Work out the finished part from the listing and answer in its coordinate system (mm). Face numbers are marked on the shaded views. A direction names the side the tool comes from. Round coordinates to 2 decimals unless told otherwise and drop trailing zeros. Write each loop counter-clockwise with the first axis right and the second up, starting at its lowest first coordinate (ties: lowest second). Pieces come first, ordered by that corner, then holes. Notation, with made-up numbers: (20.25, 14.25) - (34.25, 14.25) arc R33 cw to (34.25, 48.25) - close; hole circle Ø5 at (89.5, 16). An arc over 180 degrees is marked (long way). Answer as a JSON object with one key per item and string values.
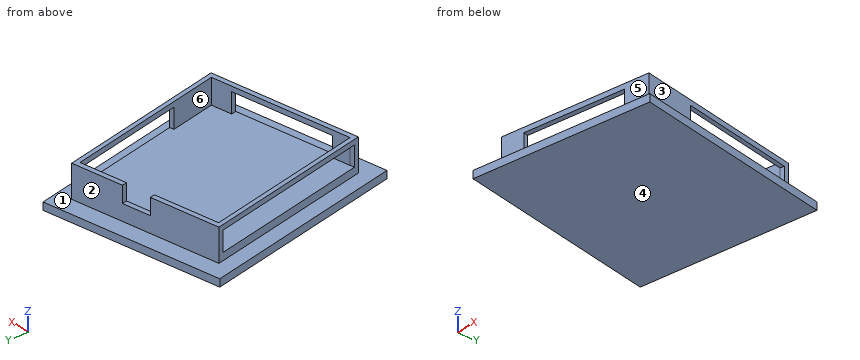
Autodesk Inventor part; units mm, degrees
ref_plane "YZ Plane" through (0, 0, 0) normal (1, 0, 0) x (0, 1, 0)
ref_plane "XZ Plane" through (0, 0, 0) normal (0, 1, 0) x (-1, 0, 0)
ref_plane "XY Plane" through (0, 0, 0) normal (0, 0, 1) x (1, 0, 0)
ref_plane "Work Plane1" through (80.3117, 823.0211, 0) normal (0, 0, 1) x (0.9814259, 0.1918418, 0)
sketch "Sketch1" plane through (80.3117, 823.0211, 0) normal (0, 0, 1) x (0.9814259, 0.1918418, 0)
  line L0 (98.9183, 339.573) -> (44.3184, 339.573)
  line L1 (44.3184, 339.573) -> (44.3184, 276.403)
  line L2 (44.3184, 276.403) -> (98.9183, 276.403)
  line L3 (98.9183, 276.403) -> (98.9183, 339.573)
  line L4 (98.9183, 339.573) -> (44.3184, 276.403)
  line L5 (42.6184, 341.488) -> (100.6184, 341.488)
  line L6 (100.6184, 341.488) -> (100.6184, 274.488)
  line L7 (100.6184, 274.488) -> (42.6184, 274.488)
  line L8 (42.6184, 274.488) -> (42.6184, 341.488)
  line L9 (42.6184, 341.488) -> (100.6184, 274.488) construction
  line L10 (100.6184, 341.488) -> (42.6184, 274.488) construction
  line L11 (98.9183, 339.573) -> (44.3184, 339.573)
  line L12 (44.3184, 339.573) -> (44.3184, 276.403)
  line L13 (44.3184, 276.403) -> (98.9183, 276.403)
  line L14 (98.9183, 276.403) -> (98.9183, 339.573)
  line L15 (98.9183, 339.573) -> (44.3184, 276.403)
  line L16 (42.6184, 341.488) -> (100.6184, 341.488)
  line L17 (100.6184, 341.488) -> (100.6184, 274.488)
  line L18 (100.6184, 274.488) -> (42.6184, 274.488)
  line L19 (42.6184, 274.488) -> (42.6184, 341.488)
  line L20 (42.6184, 341.488) -> (100.6184, 274.488) construction
  line L21 (100.6184, 341.488) -> (42.6184, 274.488) construction
  point P0 (-236.7099, -792.3271)
  point P1 (71.6184, 307.988)
  point P2 (0, 0)
  point P3 (71.6184, 307.988)
  dimension "d0" = 58
  dimension "d1" = 67
  dimension "d2" = 58
  dimension "d3" = 67
sketch "Sketch2" plane through (80.3117, 823.0211, 0) normal (0, 0, 1) x (0.9814259, 0.1918418, 0)
  line L0 (98.9183, 339.573) -> (44.3184, 339.573)
  line L1 (44.3184, 339.573) -> (44.3184, 276.403)
  line L2 (44.3184, 276.403) -> (98.9183, 276.403)
  line L3 (98.9183, 276.403) -> (98.9183, 339.573)
  line L4 (42.6184, 341.488) -> (100.6184, 341.488)
  line L5 (100.6184, 341.488) -> (100.6184, 274.488)
  line L6 (100.6184, 274.488) -> (42.6184, 274.488)
  line L7 (42.6184, 274.488) -> (42.6184, 341.488)
  line L8 (42.6184, 341.488) -> (100.6184, 274.488) construction
  line L9 (100.6184, 341.488) -> (42.6184, 274.488) construction
  line L10 (98.9183, 339.573) -> (44.3184, 339.573)
  line L11 (44.3184, 339.573) -> (44.3184, 276.403)
  line L12 (44.3184, 276.403) -> (98.9183, 276.403)
  line L13 (98.9183, 276.403) -> (98.9183, 339.573)
  line L14 (42.6184, 341.488) -> (100.6184, 341.488)
  line L15 (100.6184, 341.488) -> (100.6184, 274.488)
  line L16 (100.6184, 274.488) -> (42.6184, 274.488)
  line L17 (42.6184, 274.488) -> (42.6184, 341.488)
  line L18 (42.6184, 341.488) -> (100.6184, 274.488) construction
  line L19 (100.6184, 341.488) -> (42.6184, 274.488) construction
  point P0 (-236.7099, -792.3271)
  point P1 (0, 0)
  point P2 (71.6184, 307.988)
  point P3 (0, 0)
  point P4 (71.6184, 307.988)
  dimension "d4" = 58
  dimension "d5" = 67
  dimension "d6" = 58
  dimension "d7" = 67
extrude "Extrusion1" add sketch "Sketch1" along normal blind 10
extrude "Extrusion3" add sketch "Sketch2" against normal blind 3 contours L3 L2 L1 L0 | L4 L5 L6 L7
sketch "Sketch4" plane through (69.4802, 1100.5867, -3) normal (-0.9814259, -0.1918418, 0) x (0, 0, 1)
  line L0 (3, 65.085) -> (13, 65.085)
  line L1 (3, 1.915) -> (13, 1.915)
  line L2 (3, 65.085) -> (11, 65.085)
  line L3 (11, 65.085) -> (11, 1.915)
  line L4 (11, 1.915) -> (3, 1.915)
  line L5 (3, 1.915) -> (3, 65.085)
  point P0 (3, -1066.8151)
  dimension "d14" = 8
extrude "Extrusion4" cut sketch "Sketch4" against normal blind 3
sketch "Sketch5" plane through (126.4029, 1111.7135, -3) normal (0.1918418, -0.9814259, 0) x (0.9814259, 0.1918418, 0)
  line L0 (-56.3, 5) -> (-56.3, 3)
  line L1 (-41.56, 9.2) -> (-44.06, 9.2)
  line L2 (-14.575, 10) -> (-14.575, 9.2)
  line L3 (-9.7, 11) -> (-9.7, 3)
  line L4 (-46.3, 11) -> (-9.7, 11)
  line L5 (-9.7, 3) -> (-46.3, 3)
  line L6 (-58, 3) -> (-1.7, 3)
  line L7 (-46.3, 11) -> (-43.3, 11)
  line L8 (-43.3, 3) -> (-46.3, 3)
  line L9 (-46.3, 11) -> (-49.3, 11)
  line L10 (-49.3, 11) -> (-49.3, 3)
  line L11 (-49.3, 3) -> (-46.3, 3)
  point P0 (-337.3282, 3)
  dimension "d22" = 8
  dimension "d24" = 8
  dimension "d33" = 3
  dimension "d34" = 3
extrude "Extrusion5" cut sketch "Sketch5" against normal blind 3
sketch "Sketch6" plane through (113.5495, 1177.4691, 10) normal (0.9814259, 0.1918418, 0) x (0, 0, -1)
  line L0 (8, -44.46) -> (3, -44.46)
  line L1 (2, -65.085) -> (2, -1.915)
  line L2 (2, -65.085) -> (10, -65.085)
  line L3 (10, -65.085) -> (10, -47.085)
  line L4 (10, -47.085) -> (2, -47.085)
  line L5 (2, -47.085) -> (2, -65.085)
  line L6 (10, -65.085) -> (10, -1.915)
  line L7 (2, -47.085) -> (10, -47.085)
  line L8 (10, -47.085) -> (10, -1.915)
  line L9 (10, -1.915) -> (2, -1.915)
  line L10 (2, -1.915) -> (2, -47.085)
  point P0 (10, -1133.8151)
  dimension "d25" = 8
  dimension "d26" = 18
extrude "Extrusion6" cut sketch "Sketch6" against normal blind 3 contours L1 L9 L6 L4
sketch "Sketch7" plane through (56.9942, 1164.4628, 0) normal (0.1918418, -0.9814259, 0) x (0.9814259, 0.1918418, 0)
  line L0 (28.4907, 10.1469) -> (28.4907, 10.1469)
  line L1 (27, 8) -> (27, 3.4394)
  line L2 (27, 3.4394) -> (38, 3.4394)
  line L3 (38, 3.4394) -> (38, 8)
  line L4 (38, 3.4394) -> (27, 3.4394)
  line L5 (27, 3.4394) -> (27, 13.4394)
  line L6 (27, 13.4394) -> (38, 13.4394)
  line L7 (38, 13.4394) -> (38, 3.4394)
  point P0 (-279.3282, 0)
  point P1 (35.9907, 10.1469)
  dimension "d29" = 11
  dimension "d32" = 10
extrude "Extrusion7" cut sketch "Sketch7" against normal blind 3
sketch "Sketch8" plane through (80.3117, 823.0211, -3) normal (0, 0, -1) x (-0.9814259, -0.1918418, 0)
  line L0 (-42.6184, 341.488) -> (-100.6184, 341.488)
  line L1 (-100.6184, 341.488) -> (-100.6184, 274.488)
  line L2 (-42.6184, 274.488) -> (-42.6184, 341.488)
  line L3 (-100.6184, 274.488) -> (-42.6184, 274.488)
  line L4 (-106.4184, 348.188) -> (-36.8184, 348.188)
  line L5 (-36.8184, 348.188) -> (-36.8184, 267.788)
  line L6 (-36.8184, 267.788) -> (-106.4184, 267.788)
  line L7 (-106.4184, 267.788) -> (-106.4184, 348.188)
  point P0 (236.7099, -792.3271)
  point P1 (-71.6184, 341.488)
  point P2 (-71.6184, 307.988)
extrude "Extrusion8" add sketch "Sketch8" along normal blind 3 contours L2 L3 L1 L0 | L4 L5 L6 L7
properties part number "Syno"
Item 1: A cutting plane is placed at D-D (x = 89). Write down the section's boundary in (y, z), and give its area (3 significant figures).
Results found:
{"outline": "(1097.58, -6) - (1179.5, -6) - (1179.5, -3) - (1172.67, -3) - (1172.67, 3.44) - (1170.72, 3.44) - (1170.72, 0) - (1104.4, 0) - (1104.4, -3) - (1097.58, -3) - close; (1104.4, 8) - (1106.35, 8) - (1106.35, 10) - (1104.4, 10) - close", "area": "461 mm²"}
Item 2: For the marked faces 1, 2 and 3, determine the directions among +Z, -Z, +X, -X, +Y, -Y from which every point of the face is accessible in a straight line to the end or side of a thin tool.
Results found:
{"face 1": "+Z", "face 2": "+Z, -X, +Y", "face 3": "+Z, +X, +Y"}
Item 3: Consider line 1 along Z through (x, y) = (61.5, 1173); line 2 along Z through (x, y) = (82, 1122); line 3 along Y through (x, z) = (76, 8). Determine where each line is inside the solid, lowest interval first.
Results found:
{"line 1": "-6 to -3", "line 2": "-6 to 0", "line 3": "1101.86 to 1103.81, 1168.18 to 1170.13"}
Item 4: A cutting plane is placed at C-C (x = 74.5). Write down the section's boundary in (y, z), and give its area (3 significant figures).
Results found:
{"outline": "(1094.74, -6) - (1176.66, -6) - (1176.66, -3) - (1169.84, -3) - (1169.84, 10) - (1167.88, 10) - (1167.88, 0) - (1103.52, 0) - (1103.52, 10) - (1101.57, 10) - (1101.57, -3) - (1094.74, -3) - close", "area": "490 mm²"}
Item 5: Determine the mould class of the marked faces 4, 5 and 6 for opening direction Y: pulls with the +Y half, pulls with the -Y half, needs draft (parallel to the pull), parting line crosses it, or undercut.
Results found:
{"face 4": "needs draft", "face 5": "pulls with the -Y half", "face 6": "undercut"}
Item 6: Each of these flat-tipped pins is pushed along its axis until it touches: P1, Ø6, axis at y = 1142, z = -4, coming from the -X side; P2, Ø6, axis at x = 83.5, z = -2, coming from the +Y side; P3, Ø1, axis at x = 103.5, z = 1.5, coming from the +Y side. Where does it stop, or does it pass through?
Results found:
{"P1": "x = 54.89", "P2": "y = 1178.97", "P3": "y = 1175.6"}
Item 7: A cutting plane is placed at A-A (x = 63). Write down the section's boundary in (y, z).
Results found:
{"outline": "(1103.51, -6) - (1174.41, -6) - (1174.41, -3) - (1167.59, -3) - (1167.59, 10) - (1165.64, 10) - (1165.64, 0) - (1133.74, 0) - (1133.74, -3) - (1103.51, -3) - close; (1133.74, 8) - (1142.6, 8) - (1142.6, 10) - (1133.74, 10) - close"}
Item 8: A cutting plane is placed at B-B (y = 1148). Write down the section's boundary in (x, z).
Results found:
{"outline": "(54.3, -6) - (125.22, -6) - (125.22, -3) - (119.31, -3) - (119.31, 0) - (60.21, 0) - (60.21, -3) - (54.3, -3) - close; (60.21, 8) - (61.94, 8) - (61.94, 10) - (60.21, 10) - close; (117.58, 8) - (119.31, 8) - (119.31, 10) - (117.58, 10) - close"}
